Geometry: final body of the model. Coordinates: model frame, mm. A direction names the side the tool comes from. Give positions to 0.01 mm unless a question says otherwise; leave off trailing zeros. Loops run counter-clockwise (first coordinate to the right, second up) from the corner with the lowest first, then second, coordinate; pieces in that order, holes last.
from build123d import *

# Parameters (mm, degrees)
F1_DEPTH    = 25.4
F3_DEPTH    = 25.4
F5_DEPTH    = 25.4
F6_T1_DEPTH = 92.8531269327
F7_R        = 5.5593746135
F8_DEPTH    = 25.4
F9_R        = 5.8665873172
F10_DEPTH   = 25.4
F9_R_2      = 5.7482740473
F11_DEPTH   = 25.4


# Not quite as in the source:
# - a fillet or chamfer that OpenCascade refuses, or shapes differently, is made with other operations: its cross-section is extruded or revolved along the edge and cut away or added


with BuildPart() as f1:
    # F0 (on Front) → F1 (new body)
    with BuildSketch(Plane.XZ):
        Polygon((25.4, 12.7), (0, 12.7), (0, 0), (76.2, 0), (76.2, 12.7), (50.8, 12.7), (50.8, 38.1), (25.4, 38.1), align=None)
    extrude(amount=F1_DEPTH)

    # F2 (on face) → F3 (cut)
    with BuildSketch(Plane.XY.offset(12.7)):
        with BuildLine():
            ThreePointArc((0, -10.3920384811), (2.632385222, -4.2752682762), (7.7379127033, 0))
            Line((7.7379127033, 0), (0, 0))
            Line((0, 0), (0, -10.3920384811))
        make_face()
        with BuildLine():
            ThreePointArc((7.1188798174, -25.4), (2.4265465189, -21.1696188601), (0, -15.3364389071))
            Line((0, -15.3364389071), (0, -25.4))
            Line((0, -25.4), (7.1188798174, -25.4))
        make_face()
    extrude(amount=-F3_DEPTH, mode=Mode.SUBTRACT)

    # F4 (on face) → F5 (cut)
    with BuildSketch(Plane.XY.offset(12.7)):
        with BuildLine():
            ThreePointArc((68.4031397104, 0), (73.7378443896, -4.7264477616), (76.2, -11.4149582241))
            Line((76.2, -11.4149582241), (76.2, 0))
            Line((76.2, 0), (68.4031397104, 0))
        make_face()
        with BuildLine():
            ThreePointArc((76.2, -14.5105812124), (74.030690178, -20.7530692397), (69.3316906691, -25.4))
            Line((69.3316906691, -25.4), (76.2, -25.4))
            Line((76.2, -25.4), (76.2, -14.5105812124))
        make_face()
    extrude(amount=-F5_DEPTH, mode=Mode.SUBTRACT)

    # F6: fillet of radius 13.4906253865 on 2 edges, made by hand

    # F6_s2 → F6_t1 (cut)
    with BuildSketch(Plane.YZ.offset(-8.3265634664)):
        with BuildLine():
            ThreePointArc((-25.4, 24.6093746135), (-21.4486873067, 34.1486873067), (-11.9093746135, 38.1))
            Line((-11.9093746135, 38.1), (-25.4, 38.1))
            Line((-25.4, 38.1), (-25.4, 24.6093746135))
        make_face()
        with BuildLine():
            ThreePointArc((0, 24.6093746135), (-3.9513126933, 34.1486873067), (-13.4906253865, 38.1))
            Line((-13.4906253865, 38.1), (0, 38.1))
            Line((0, 38.1), (0, 24.6093746135))
        make_face()
    extrude(amount=F6_T1_DEPTH, mode=Mode.SUBTRACT)

    # F7 (on face) → F8 (cut)
    with BuildSketch(Plane.YZ.offset(50.8)):
        with Locations((-11.9093746135, 24.6093746135)):
            Circle(F7_R)
    extrude(amount=-F8_DEPTH, mode=Mode.SUBTRACT)

    # F9 (on face) → F10 (cut)
    with BuildSketch(Plane.XY.offset(12.7)):
        with Locations((62.5223219395, -12.8642386941)):
            Circle(F9_R)
    extrude(amount=-F10_DEPTH, mode=Mode.SUBTRACT)

    # F9 (on face) → F11 (cut)
    with BuildSketch(Plane.XY.offset(12.7)):
        with Locations((14.1673966027, -12.8642386941)):
            Circle(F9_R_2)
    extrude(amount=-F11_DEPTH, mode=Mode.SUBTRACT)


solid = f1.part
Item 1: Section query C-C on y = -5. Return loops of the section in (x, z), plus the area to 3 significant figures.
Values follow:
outline: (2.13, 0) - (73.92, 0) - (73.92, 12.7) - (50.8, 12.7) - (50.8, 35.09) - (25.4, 35.09) - (25.4, 12.7) - (2.13, 12.7) - close
area: 1,480 mm2
Item 2: Pin query (flat end, axial travel): pin 1 (7 mm diameter, centred on x = 62.52, y = -12.86, fed in from +Z); pin 2 (6 mm diameter, centred on x = 28.5, z = 26.5, fed in from +Y); pin 3 (5 mm diameter, centred on x = 43, y = -22.5, fed in from +Z); pin 4 (12.5 mm diameter, centred on x = 65.5, y = -16, fed in from +Z). Return the tip coordinate at first contact, or that it passes through.
Values follow:
pin 1: passes through
pin 2: stops at y = 0
pin 3: stops at z = 35.4
pin 4: stops at z = 12.7
Item 3: Set-up query: faces 4 (the face through (37.92, -21.82, 33.76)), 5 (the face through (25.4, -15.3, 19.9)), 6 (the face through (50.8, -15.3, 19.6)). Return all of +Z, -Z, +X, -X, +Y, -Y with unobstructed straight access to the full face (end or side cutting, diameter ignored); none if empty.
Values follow:
face 4: +Z, +X, -X, -Y
face 5: +Z, -X, +Y, -Y
face 6: +Z, +X, +Y, -Y
Item 4: Section query D-D on z = 2.5. Return loops of the section in (x, y).
Values follow:
outline: (0, -15.34) arc R14.38 ccw to (7.12, -25.4) - (69.33, -25.4) arc R14.6 ccw to (76.2, -14.51) - (76.2, -11.41) arc R14.6 ccw to (68.4, 0) - (7.74, 0) arc R14.38 ccw to (0, -10.39) - close; hole circle Ø11.5 at (14.17, -12.86); hole circle Ø11.73 at (62.52, -12.86)
Item 5: Section query A-A on x = 50. Return loops of the section in (y, z), plus the area to 3 significant figures.
Values follow:
outline: (-25.4, 0) - (0, 0) - (0, 24.61) arc R13.49 ccw to (-12.7, 38.08) arc R13.49 ccw to (-25.4, 24.61) - close; hole circle Ø11.12 at (-11.91, 24.61)
area: 793 mm2
Item 6: Section query B-B on z = 21.5. Return loops of the section in (x, y), plus the area to 3 significant figures.
Values follow:
outline: (25.4, -25.4) - (50.8, -25.4) - (50.8, -16.52) - (25.4, -16.52) - close; (25.4, -7.3) - (50.8, -7.3) - (50.8, 0) - (25.4, 0) - close
area: 411 mm2
Item 7: Ray query, probe 1 along X at (y, z) = (-13, 8); probe 2 along X at (y, z) = (-11.5, 10); probe 3 along Z at (x, y) = (21, -12.25). Return the intervals inside material, ascending.
Values follow:
probe 1: x = 0 to 8.42, 19.91 to 56.66, 68.39 to 76.2
probe 2: x = 0 to 8.58, 19.75 to 56.82, 68.23 to 76.2
probe 3: z = 0 to 12.7
Item 8: Draft query along Z for faces 1 (the face through (0, -13, 6)), 2 (the face through (13, -7, 12.7)), 3 (the face through (38.28, -13.11, 19.18)). Return one class per face: +Z half, -Z half, draft (parallel to the pull), parting line (faces both ways), or undercut.
Values follow:
face 1: draft
face 2: +Z half
face 3: undercut
